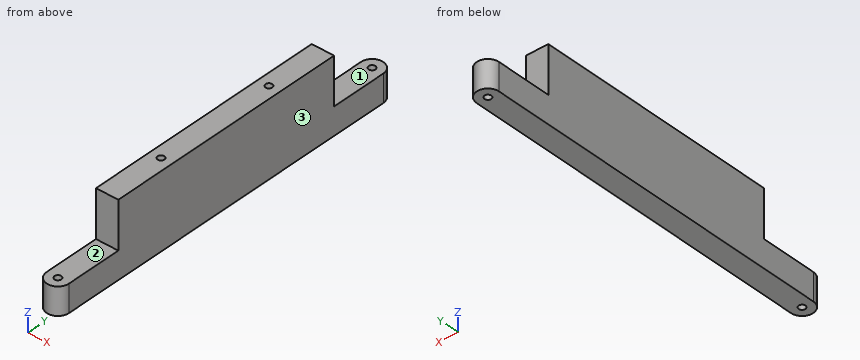
```python
from build123d import *

# Parameters (mm, degrees)
SKETCH_1_R          = 2
SKETCH_1_R_2        = 0.6
EXTRUDE_1_DEPTH     = 20
SKETCH_4_W          = 4
SKETCH_4_H          = 20
EXTRUDE_2_DEPTH     = 10
SKETCH_3_W          = 4
SKETCH_3_H          = 10.2
CUT_EXTRUDE_1_DEPTH = 24.409399821
EXTRUDE_START       = 10
SKETCH_4_2_W        = 4
SKETCH_4_2_H        = 20
EXTRUDE_3_DEPTH     = 3
SKETCH_1_4_R        = 0.6
CUT_EXTRUDE_3_DEPTH = 24.937418407
SKETCH_5_W          = 4
SKETCH_5_H          = 18.9
EXTRUDE_4_DEPTH     = 20
SKETCH_6_W          = 6.65
SKETCH_6_H          = 67.8
CUT_EXTRUDE_4_DEPTH = 69.888605734
SKETCH_7_R          = 0.6
CUT_EXTRUDE_5_DEPTH = 3


with BuildPart() as part:
    # Sketch 1 → Extrude 1 (new body)
    with BuildSketch(Plane.XY):
        Circle(SKETCH_1_R)
        Circle(SKETCH_1_R_2, mode=Mode.SUBTRACT)
    extrude(amount=EXTRUDE_1_DEPTH)

    # Sketch 4 → Extrude 2 (add)
    with BuildSketch(Plane(origin=(0, 0, 0), x_dir=(1, 0, 0), z_dir=(0, 1, 0))):
        with Locations((0, -10)):
            Rectangle(SKETCH_4_W, SKETCH_4_H)
    extrude(amount=EXTRUDE_2_DEPTH)

    # Sketch 3 → Cut-Extrude 1 (cut, through all)
    with BuildSketch(Plane(origin=(0, 10, 0), x_dir=(1, 0, 0), z_dir=(0, 1, 0))):
        with Locations((0, -10)):
            Rectangle(SKETCH_3_W, SKETCH_3_H)
    extrude(amount=-CUT_EXTRUDE_1_DEPTH, mode=Mode.SUBTRACT)


with BuildPart() as cut_extrude_1_piece_1:
    # of the separate pieces the step leaves, piece 1, a body of its own (cut_extrude_1_pieces)
    add(part.part.solids().sort_by_distance((-2, 0, 0))[0])



with BuildPart() as cut_extrude_1_piece_2:
    # of the separate pieces the step leaves, piece 2, a body of its own (cut_extrude_1_pieces)
    add(part.part.solids().sort_by_distance((2, 0, 15.1))[0])


with BuildPart() as cut_extrude_1_piece_1_1:
    add(cut_extrude_1_piece_1.part)

    add(cut_extrude_1_piece_2.part)  # Extrude 3 merges Cut-Extrude 1 piece 2
    # Sketch 4_2 → Extrude 3 (add)
    with BuildSketch(Plane(origin=(0, 0, 0), x_dir=(1, 0, 0), z_dir=(0, 1, 0)).offset(EXTRUDE_START)):
        with Locations((0, -10)):
            Rectangle(SKETCH_4_2_W, SKETCH_4_2_H)
    extrude(amount=EXTRUDE_3_DEPTH)

    # Sketch 1_4 → Cut-Extrude 3 (cut, through all)
    with BuildSketch(Plane.XY):
        with Locations(Location((0, 0, 0), (0, 0, 180))):
            Circle(SKETCH_1_4_R)
    extrude(amount=CUT_EXTRUDE_3_DEPTH, mode=Mode.SUBTRACT)

    # Sketch 5 → Extrude 4 (add)
    with BuildSketch(Plane(origin=(0, 0, 0), x_dir=(-1, 0, 0), z_dir=(0, 0, -1))):
        with Locations((0, 22.45)):
            Rectangle(SKETCH_5_W, SKETCH_5_H)
    extrude(amount=-EXTRUDE_4_DEPTH)

    # Mirror 1: Cut-Extrude 1 piece 1 across plane


with BuildPart() as cut_extrude_1_piece_1_2:
    add(cut_extrude_1_piece_1_1.part)
    add(cut_extrude_1_piece_1_1.part.mirror(Plane(origin=(2, 31.9, 39.318643845), x_dir=(0, 0, 1), z_dir=(0, 1, 0))))

    # Sketch 6 → Cut-Extrude 4 (cut, through all)
    with BuildSketch(Plane.ZY.offset(2)):
        with Locations((16.675, 31.9)):
            Rectangle(SKETCH_6_W, SKETCH_6_H)
    extrude(amount=-CUT_EXTRUDE_4_DEPTH, mode=Mode.SUBTRACT)

    # Sketch 7 → Cut-Extrude 5 (cut)
    with BuildSketch(Plane.XY.offset(13.35)):
        with Locations((0, 42.85)):
            Circle(SKETCH_7_R)
        with Locations((0, 20.95)):
            Circle(SKETCH_7_R)
    extrude(amount=-CUT_EXTRUDE_5_DEPTH, mode=Mode.SUBTRACT)


solid = cut_extrude_1_piece_1_2.part
```
Design review of the part built by this model. Coordinates are the model's own, in mm. Face numbers are marked on the shaded views. A direction names the side the tool comes from. Give positions to 0.01 mm unless a question says otherwise; leave off trailing zeros. Loops run counter-clockwise (first coordinate to the right, second up) from the corner with the lowest first, then second, coordinate; pieces in that order, holes last. Notation, with made-up numbers: (-10, 75) -> (14, 75) arc R33 cw to (14, 112) -> close; hole circle Ø7 at (-21.75, -2.5). An arc over 180 degrees is marked (long way). One line per item, written item: value.
Q1. Machinability: for the marked faces 1, 2 and 3, which of the approach directions +Z, -Z, +X, -X, +Y, -Y give a long, thin tool a straight path to every point of the face, cutting with its end or side? Answer none if there is none.
Numbers:
face 1: +Z, +X, -X, +Y
face 2: +Z, +X, -X, -Y
face 3: +Z, -Z, +X, +Y, -Y
Q2. We need section D-D on z = 4. Give the boundary of the cut face in (x, y), and give its area (3 significant figures).
Numbers:
outline: (-2, 0) arc R2 ccw to (2, 0) -> (2, 63.8) arc R2 ccw to (-2, 63.8) -> close; hole circle Ø1.2 at (0, 0); hole circle Ø1.2 at (0, 63.8)
area: 266 mm^2
Q3. For L1, parallel to Y at x = 0, z = 11.85; L2, parallel to Y at x = 0, z = 1.2; L3, parallel to X at y = 42.85, z = 11.65, list the stretches that pass through material, from the lowest coordinate up.
Numbers:
L1: y = 10 to 20.35, 21.55 to 42.25, 43.45 to 53.8
L2: y = -2 to -0.6, 0.6 to 63.2, 64.4 to 65.8
L3: x = -2 to -0.6, 0.6 to 2
Q4. For pin 1 Ø1 at (x, y) = (0, 21) entering from +Z; pin 2 Ø1.9 at (x, y) = (0, 63.8) entering from +Z; pin 3 Ø2 at (x, z) = (-1, 9.5) entering from -Y, all flat-tipped, find the tip position at first contact; note any pin that passes through.
Numbers:
pin 1: stops at z = 10.35
pin 2: stops at z = 4.9
pin 3: stops at y = 10
Q5. We need section C-C on y = 9. Give the boundary of the cut face in (x, z), and give its area (3 significant figures).
Numbers:
outline: (-2, 0) -> (2, 0) -> (2, 4.9) -> (-2, 4.9) -> close
area: 19.6 mm^2
Q6. We need section A-A on x = 0. Give the boundary of the cut face in (y, z).
Numbers:
outline: (-2, 0) -> (-0.6, 0) -> (-0.6, 4.9) -> (-2, 4.9) -> close; (0.6, 0) -> (63.2, 0) -> (63.2, 4.9) -> (53.8, 4.9) -> (53.8, 13.35) -> (43.45, 13.35) -> (43.45, 10.35) -> (42.25, 10.35) -> (42.25, 13.35) -> (21.55, 13.35) -> (21.55, 10.35) -> (20.35, 10.35) -> (20.35, 13.35) -> (10, 13.35) -> (10, 4.9) -> (0.6, 4.9) -> close; (64.4, 0) -> (65.8, 0) -> (65.8, 4.9) -> (64.4, 4.9) -> close
Q7. We need section B-B on z = 11. Give the boundary of the cut face in (x, y), and give its area (3 significant figures).
Numbers:
outline: (-2, 10) -> (2, 10) -> (2, 53.8) -> (-2, 53.8) -> close; hole circle Ø1.2 at (0, 20.95); hole circle Ø1.2 at (0, 42.85)
area: 173 mm^2
